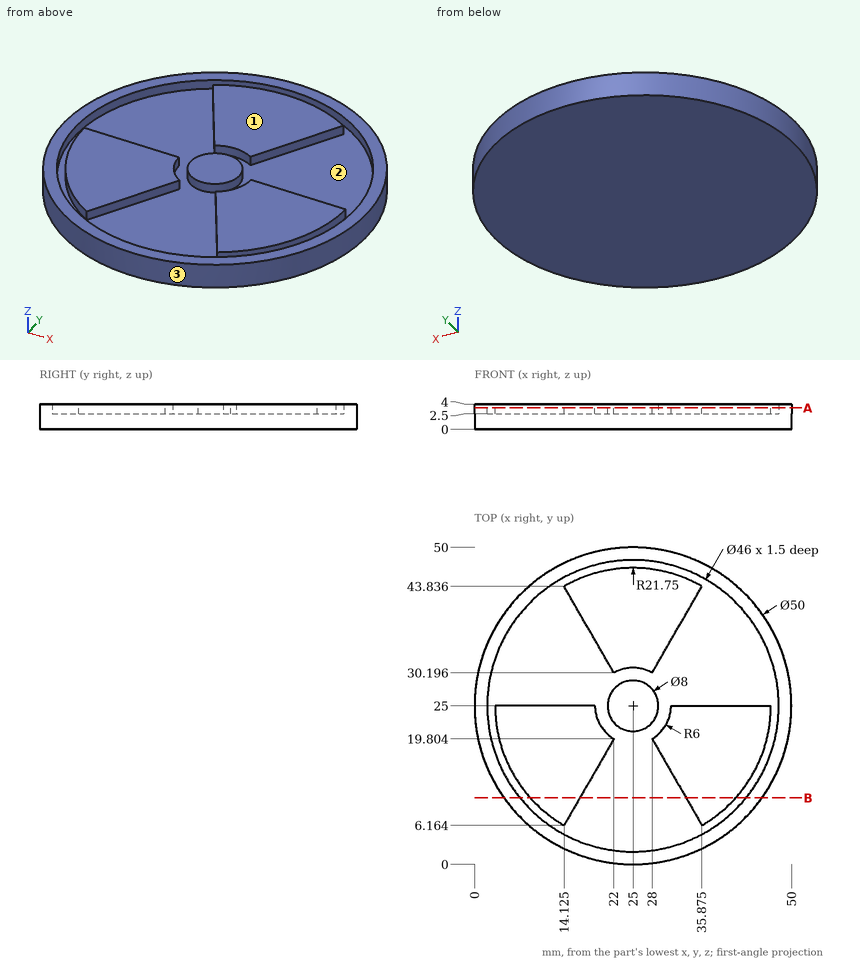
Here's the drawing with two shaded views (mm, measured from the low corner). I have some questions. Coordinates: 2 decimals unless noted, no trailing zeros. Loops run counter-clockwise (first coordinate to the right, second up) from the corner with the lowest first, then second, coordinate; pieces in that order, holes last. Notation, with made-up numbers: M 25.5,-4.5 L 35.5,-4.5 A38 cw 35.5,34.5 Z; hole C 50,68 d10. An arc over 180 degrees is marked long. Return JSON: item names as keys, results as strings. Group by question number.
Item 1: Thinking about a two-plate mould opening in Y: for the marked faces 1, 2 and 3, which applies, released by +Y, released by -Y, zero draft, split by the parting line, or undercut?
Item 2: Imagine slicing it at B-B (y = 10.5). Please give me the cut outline in (x, z), and give its area (3 significant figures).
Item 3: If I drill on L1, parallel to Y at x = 25, z = 3.35; L2, parallel to Y at x = 35, z = 3.35 (1 decimal); L3, parallel to X at y = 44, z = 3.75 (1 decimal), over which ranges is the centre line in solid material (lowest first)? Write a range as from..to.
Item 4: Imagine slicing it at A-A (z = 3.4). Give the number of separate pieces and of enclosed holes in the cut face, and give its area (3 significant figures).
Item 5: I'm going to push flat-ended pins straight in: pin 1 Ø1 at (x, y) = (21.5, 7.5) entering from -Z; pin 2 Ø1 at (y, z) = (8.5, 1.5) entering from +X; pin 3 Ø1 at (x, z) = (27.5, 2.5) entering from +Y; pin 4 Ø1.2 at (x, z) = (12, 3) entering from +Y. Where does each tip first touch, or does it pass through?
Verdict:
{
 "1": {"face 1": "zero draft", "face 2": "undercut", "face 3": "split by the parting line"},
 "2": {"outline": "M 4.63,0 L 45.37,0 L 45.37,4 L 42.85,4 L 42.85,2.5 L 41.21,2.5 L 41.21,4 L 33.37,4 L 33.37,2.5 L 16.63,2.5 L 16.63,4 L 8.79,4 L 8.79,2.5 L 7.15,2.5 L 7.15,4 L 4.63,4 Z", "area": "133 mm^2"},
 "3": {"L1": "y = 0..2, 21..29, 31..46.75, 48..50", "L2": "y = 2.1..4.3, 7.7..25, 42.3..44.3, 45.7..47.9", "L3": "x = 8.8..12, 14.4..35.6, 38..41.2"},
 "4": {"separate pieces": "5", "enclosed holes": "1", "area": "1,040 mm^2"},
 "5": {"pin 1": "stops at z = 0", "pin 2": "stops at x = 44.21", "pin 3": "stops at y = 49.92", "pin 4": "stops at y = 46.71"}
}
